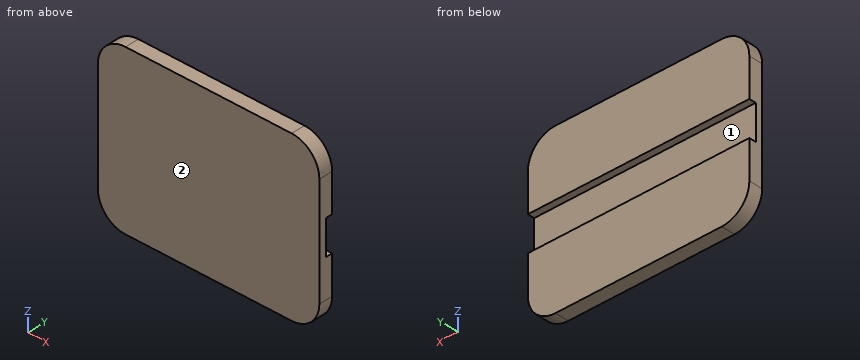
```python
from build123d import *

# Parameters (mm, degrees)
F0_W     = 160
F0_H     = 120
F2_DEPTH = 10
F1_W     = 170
F1_H     = 25
F3_DEPTH = 5
F4_R     = 20


with BuildPart() as f2:
    # F0 (on Front) → F2 (new body)
    with BuildSketch(Plane.XZ):
        Rectangle(F0_W, F0_H)
    extrude(amount=F2_DEPTH)

    # F1 (on Front) → F3 (cut)
    with BuildSketch(Plane.XZ):
        Rectangle(F1_W, F1_H)
    extrude(amount=F3_DEPTH, mode=Mode.SUBTRACT)

    # F4
    f4_edges = [f2.edges().sort_by_distance(p)[0] for p in [
        (80, -5, -60),
        (80, -5, 60),
        (-80, -5, 60),
        (-80, -5, -60),
    ]]
    fillet(f4_edges, radius=F4_R)


solid = f2.part
```
Input: part model. Units: mm. Frame: model coordinates. Face numbers are marked on the shaded views. A direction names the side the tool comes from. Give positions to 0.01 mm unless a question says otherwise; leave off trailing zeros. Write each loop counter-clockwise with the first axis right and the second up, starting at its lowest first coordinate (ties: lowest second). Pieces come first, ordered by that corner, then holes. Notation, with made-up numbers: (23.25, -24) - (30.25, -24) arc R22 cw to (30.25, -7) - close; hole circle Ø11 at (71.25, -30). An arc over 180 degrees is marked (long way). Write item = value, one per line. Start each with the question number.
1. First-contact query: pin 1 Ø4 at (y, z) = (-8.5, -46.5) entering from -X; pin 2 Ø1.5 at (y, z) = (-5.5, 43) entering from +X; pin 3 Ø1 at (x, z) = (-52, 4) entering from +Y. Flat tips, straight axial feed; report the tip coordinate or a pass-through.
2. Ray query, L1, parallel to Z at x = -5, y = -2.75; L2, parallel to Y at x = 68, z = 0.5; L3, parallel to X at y = -0.25, z = -41. Return the intervals inside material, ascending.
3. Section query C-C, the plane z = 7. Output: boundary loops of the cut face in (x, y), then the cut area to 3 significant figures.
4. Access query for the marked faces 1 and 2. Directions: +Z, -Z, +X, -X, +Y, -Y. A direction counts if a zero-diameter tool reaches every point of the face in a straight line with its end or side. Return the directions, or none.
5. Section query D-D, the plane x = -64.5. Output: boundary loops of the cut face in (y, z).
6. Section query B-B, the plane x = -10. Output: boundary loops of the cut face in (y, z).
7. Section query A-A, the plane y = -1.75. Output: boundary loops of the cut face in (x, z).
Check sheet entries:
q1.pin_1 = -79.49
q1.pin_2 = 79.87
q1.pin_3 = -5
q2.L1 = -60 to -12.5, 12.5 to 60
q2.L2 = -10 to -5
q2.L3 = -79.97 to 79.97
q3.outline = (-80, -10) - (80, -10) - (80, -5) - (-80, -5) - close
q3.area = 800 mm2
q4.face_1 = +X, -X, +Y
q4.face_2 = +Z, -Z, +X, -X, -Y
q5.outline = (-10, -59.49) - (0, -59.49) - (0, -12.5) - (-5, -12.5) - (-5, 12.5) - (0, 12.5) - (0, 59.49) - (-10, 59.49) - close
q6.outline = (-10, -60) - (0, -60) - (0, -12.5) - (-5, -12.5) - (-5, 12.5) - (0, 12.5) - (0, 60) - (-10, 60) - close
q7.outline = (-80, -40) arc R20 ccw to (-60, -60) - (60, -60) arc R20 ccw to (80, -40) - (80, -12.5) - (-80, -12.5) - close; (-80, 12.5) - (80, 12.5) - (80, 40) arc R20 ccw to (60, 60) - (-60, 60) arc R20 ccw to (-80, 40) - close
